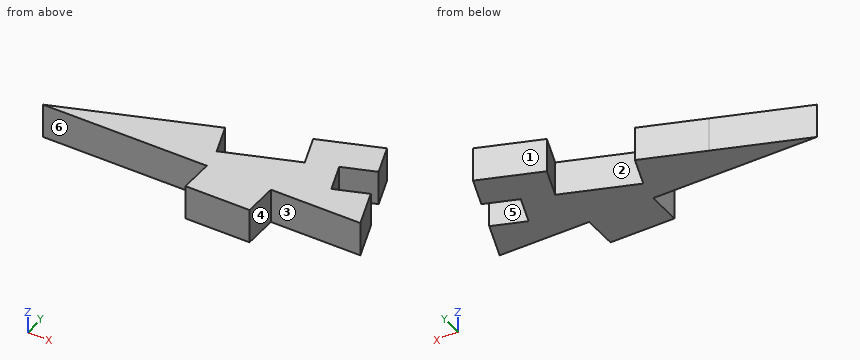
```python
from build123d import *

# Parameters (mm, degrees)
BOSS_EXTRUDE1_DEPTH = 5.08
BOSS_EXTRUDE2_DEPTH = 5.08
CUT_EXTRUDE1_DEPTH  = 6.08


with BuildPart() as part:
    # Sketch1 → Boss-Extrude1 (new body)
    with BuildSketch(Plane.XY):
        Polygon((19.624427787, 7.142707579), (8.950572213, 3.257741865), (7.213109885, 8.031380379), (-1.737462328, 4.773638514), (0, 0), (9.525, 0), (9.525, -5.08), (19.05, -5.08), (19.05, 0), (28.575, 0), (28.575, 10.400449444), (26.837537672, 15.174087958), (17.886965459, 11.916346093), align=None)
    extrude(amount=BOSS_EXTRUDE1_DEPTH)

    # Sketch2 → Boss-Extrude2 (add)
    with BuildSketch(Plane.XY.offset(5.08)):
        Polygon((28.575, 10.400449444), (28.575, 0), (32.360454021, 0), align=None)
        Polygon((0, 0), (-14.852926353, 0), (-1.737462328, 4.773638514), align=None)
    extrude(amount=-BOSS_EXTRUDE2_DEPTH)

    # Sketch3 → Cut-Extrude1 (cut, through all)
    with BuildSketch(Plane.XY.offset(5.08)):
        Polygon((28.575, 10.400449444), (30.203870933, 5.925163338), (25.430232419, 4.18770101), (23.801361486, 8.662987116), align=None)
    extrude(amount=-CUT_EXTRUDE1_DEPTH, mode=Mode.SUBTRACT)


solid = part.part
```
The listing builds one solid part. Answer for the finished solid, in the listing's coordinates (mm). Face numbers are marked on the shaded views. A direction names the side the tool comes from. Coordinates: 2 decimals unless noted, no trailing zeros. Order: outer loops, then holes, each group sorted by start corner. A loop starts at its lowest first (then second) coordinate and runs counter-clockwise, first axis right, second up. Notation, with made-up numbers: M 54,78.25 L 71,78.25 A15 cw 71,89.25 Z; hole C 26,86.5 d11. An arc over 180 degrees is marked long. Answer as a JSON object with one key per item and string values. Group by question number.
1. A tool of negligible diameter and unlimited length cuts with its end or side. For the marked faces 4, 5 and 6, from which of +Z, -Z, +X, -X, +Y, -Y can it reach the whole face along a straight path? Write none if from no direction.
2. Section A-A on z = 3.9 is taken. Write down the section's boundary in (x, y) (3 decimals), then the cut area to 3 significant figures.
3. Determine the mould class of the marked faces 1, 2 and 3 for opening direction X: released by +X, released by -X, zero draft, split by the parting line, or undercut.
4. Section C-C on y = 12.5 is taken. Write down the section's boundary in (x, z).
5. Section B-B on x = 6.5 is taken. Write down the section's boundary in (y, z), then the cut area to 3 significant figures.
6. Flat-ended cylindrical pins translate along their axes: P1, Ø2, axis at x = 14.5, z = 4, coming from the +Y side; P2, Ø3, axis at y = 12, z = 2, coming from the -X side; P3, Ø2.5, axis at x = -6.5, z = 2, coming from the -Y side. Find the tip coordinate at first contact, or state that the pin passes through.
7. Straight lines are drawn through the part: line 1 (X direction, y = -3.75, z = 2.15) (3 decimals); line 2 (X direction, y = 11.5, z = 2.8); line 3 (Y direction, x = -9.5, z = 2.95). For each, find the intervals that lie inside material, in ascending order.
Values follow:
{
 "1": {"face 4": "+Z, -Z, +X, -Y", "face 5": "+Z, -Z", "face 6": "+Z, -Z, -X, -Y"},
 "2": {"outline": "M -14.853,0 L 9.525,0 L 9.525,-5.08 L 19.05,-5.08 L 19.05,0 L 32.36,0 L 30.204,5.925 L 25.43,4.188 L 23.801,8.663 L 28.575,10.4 L 26.838,15.174 L 17.887,11.916 L 19.624,7.143 L 8.951,3.258 L 7.213,8.031 Z", "area": "325 mm2"},
 "3": {"face 1": "released by -X", "face 2": "undercut", "face 3": "zero draft"},
 "4": {"outline": "M 19.49,0 L 27.81,0 L 27.81,5.08 L 19.49,5.08 Z"},
 "5": {"outline": "M 0,0 L 7.77,0 L 7.77,5.08 L 0,5.08 Z", "area": "39.5 mm2"},
 "6": {"P1": "y = 5.64", "P2": "x = 17.89", "P3": "y = 0"},
 "7": {"line 1": "9.525 to 19.05", "line 2": "18.04 to 28.17", "line 3": "0 to 1.95"}
}
